Geometry: see drawing. Coordinates: mm, zero at the bounding-box minimum. Round coordinates to 2 decimals unless told otherwise and drop trailing zeros. Write each loop counter-clockwise with the first axis right and the second up, starting at its lowest first coordinate (ties: lowest second). Pieces come first, ordered by that corner, then holes. Notation, with made-up numbers: M 24,9 L 31,9 A16 cw 31,14 Z; hole C -17.5,-5.5 d7. An arc over 180 degrees is marked long. Write each question's results on one line, items separated by ' | '. Start each with the question number.
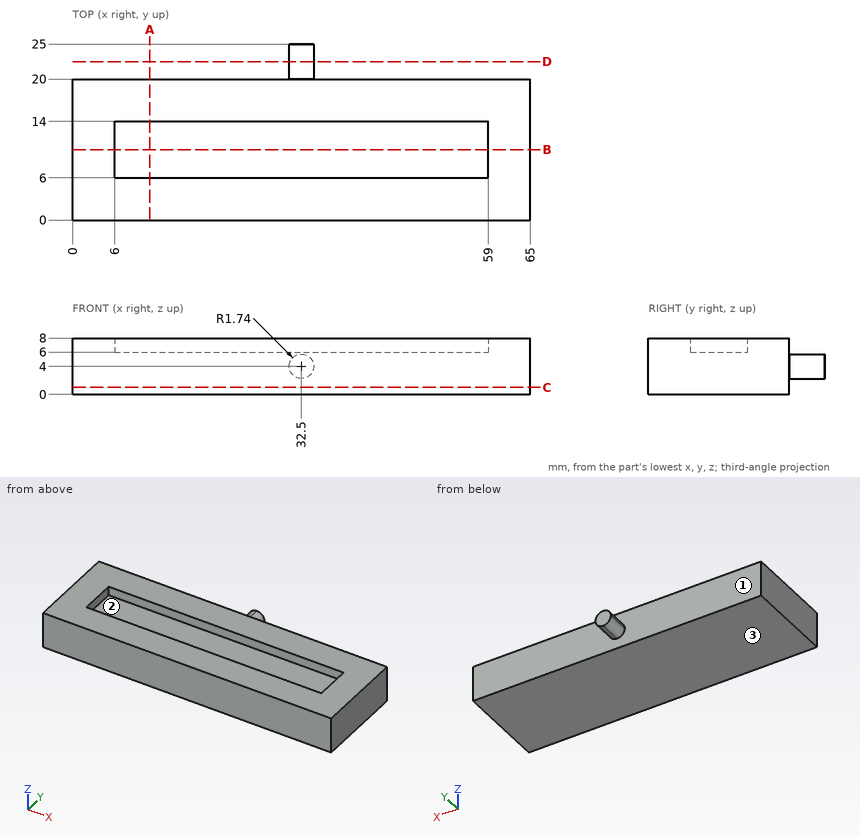
1. Line query: L1, parallel to Y at x = 24.5, z = 7; L2, parallel to X at y = 8, z = 7.25; L3, parallel to Z at x = 13, y = 11.5. Output: solid intervals per line, ascending. Write a range as from..to.
2. Cut plane A-A on x = 11. Output: boundary loops of the cut face in (y, z), and give its area (3 significant figures).
3. Cut plane C-C on z = 1. Output: boundary loops of the cut face in (x, y).
4. Contact query for flat-ended pins moving along their axis: P1, Ø4, axis at y = 4, z = 7, coming from the -X side; P2, Ø4, axis at x = 45, z = 4.5, coming from the +Y side. Output: stop coordinate, or through.
5. Cut plane B-B on y = 10. Output: boundary loops of the cut face in (x, z), and give its area (3 significant figures).
6. Draft query along Y for the marked faces 1, 2 and 3. Return one class per face: +Y half, -Y half, draft (parallel to the pull), parting line (faces both ways), or undercut.
7. Cut plane D-D on y = 22.5. Output: boundary loops of the cut face in (x, z).
Answers follow:
1) L1: y = 0..6, 14..20 | L2: x = 0..6, 59..65 | L3: z = 0..6
2) outline: M 0,0 L 20,0 L 20,8 L 14,8 L 14,6 L 6,6 L 6,8 L 0,8 Z | area: 144 mm2
3) outline: M 0,0 L 65,0 L 65,20 L 0,20 Z
4) P1: stops at x = 0 | P2: stops at y = 20
5) outline: M 0,0 L 65,0 L 65,8 L 59,8 L 59,6 L 6,6 L 6,8 L 0,8 Z | area: 414 mm2
6) face 1: +Y half | face 2: undercut | face 3: draft
7) outline: C 32.5,4 d3.48
